Check sheet for the drawn part. Datum: minimum x, y, z corner. Units: mm. A direction names the side the tool comes from. Coordinates: 2 decimals unless noted, no trailing zeros. Order: outer loops, then holes, each group sorted by start corner. A loop starts at its lowest first (then second) coordinate and runs counter-clockwise, first axis right, second up. Notation, with made-up numbers: (10.5, 15.25) -> (23.5, 15.25) arc R26 cw to (23.5, 29.25) -> close; hole circle Ø4 at (-37.5, 64.5). An arc over 180 degrees is marked (long way). Answer as CSV lines item,"result".
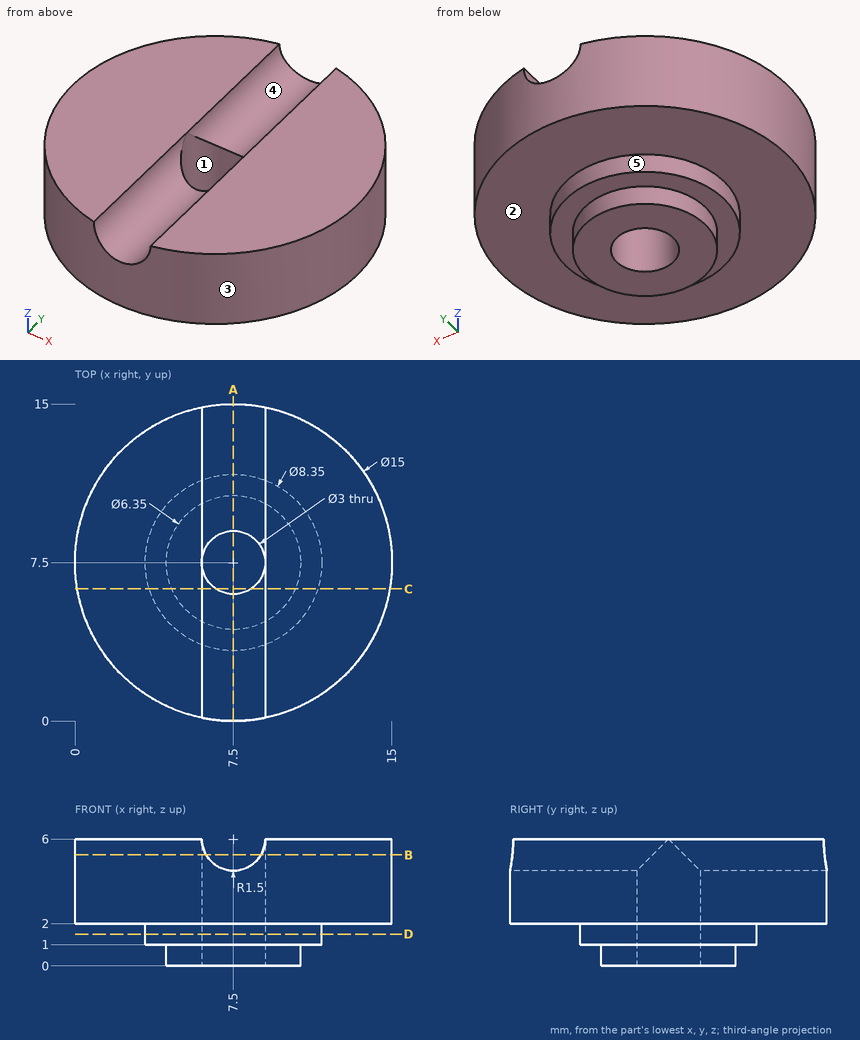
Item 1: Thickness scan on line 1 (Y direction, x = 7.5, z = 2.9); line 2 (Z direction, x = 3, y = 4); line 3 (Y direction, x = 7.75, z = 0.75). Record the ranges inside material, lowest first.
Answer list:
line 1,"0 to 6, 9 to 15"
line 2,"2 to 6"
line 3,"4.33 to 6.02, 8.98 to 10.67"
Item 2: Section check B-B, the plane z = 5.25. Record the boundary of the cut face in (x, y).
Answer list:
outline,"(6.2, 0.11) -> (6.2, 6.75) arc R1.5 cw to (6.2, 8.25) -> (6.2, 14.89) arc R7.5 ccw to start; (8.8, 0.11) arc R7.5 ccw to (8.8, 14.89) -> (8.8, 8.25) arc R1.5 cw to (8.8, 6.75) -> close"
Item 3: Section check C-C, the plane y = 6.25. Record the boundary of the cut face in (x, z).
Answer list:
outline,"(0.1, 2) -> (3.52, 2) -> (3.52, 1) -> (4.58, 1) -> (4.58, 0) -> (6.67, 0) -> (6.67, 4.75) arc R1.5 cw to (6, 6) -> (0.1, 6) -> close; (8.33, 0) -> (10.42, 0) -> (10.42, 1) -> (11.48, 1) -> (11.48, 2) -> (14.9, 2) -> (14.9, 6) -> (9, 6) arc R1.5 cw to (8.33, 4.75) -> close"
Item 4: Depth check by flat-ended pin: pin 1 Ø1 at (x, z) = (13, 3) entering from +Y; pin 2 Ø3 at (y, z) = (12, 3.5) entering from -X; pin 3 Ø1.5 at (y, z) = (6, 2) entering from +X. Enter the tip coordinate at first touch or a pass-through.
Answer list:
pin 1,"y = 13.09"
pin 2,"x = 0.63"
pin 3,"x = 14.96"
Item 5: Section check D-D, the plane z = 1.5. Record the boundary of the cut face in (x, y) (3 decimals), plus the area to 3 significant figures.
Answer list:
outline,"circle Ø8.35 at (7.5, 7.5); hole circle Ø3 at (7.5, 7.5)"
area,"47.7 mm2"
Item 6: Tool access check on the marked faces 4 and 5. Record the directions out of +Z, -Z, +X, -X, +Y, -Y that give a thin tool (end or side, any length) a straight path to the whole face; none if there is none.
Answer list:
face 4,"+Z, +Y, -Y"
face 5,"-Z"
Item 7: Release check for a two-part mould opening along X. For the marked faces 1, 2 and 3 record: +X half, -X half, draft (parallel to the pull), parting line (faces both ways), or undercut.
Answer list:
face 1,"undercut"
face 2,"draft"
face 3,"parting line"
Item 8: Section check A-A, the plane x = 7.5. Record the boundary of the cut face in (y, z) (3 decimals).
Answer list:
outline,"(0, 2) -> (3.325, 2) -> (3.325, 1) -> (4.325, 1) -> (4.325, 0) -> (6, 0) -> (6, 4.5) -> (0, 4.5) -> close; (9, 0) -> (10.675, 0) -> (10.675, 1) -> (11.675, 1) -> (11.675, 2) -> (15, 2) -> (15, 4.5) -> (9, 4.5) -> close"
